Check sheet for the modelled part. Datum: model origin and axes. Units: mm. Give positions to 0.01 mm unless a question says otherwise; leave off trailing zeros. Order: outer loops, then holes, each group sorted by start corner. A loop starts at its lowest first (then second) coordinate and runs counter-clockwise, first axis right, second up. Notation, with made-up numbers: (-33.5, 8) -> (19.5, 8) arc R18 cw to (19.5, 27) -> close; hole circle Ø4 at (32, -34.5). An arc over 180 degrees is marked (long way). One line per question, with ' | ' between items.
```python
from build123d import *

# Parameters (mm, degrees)
SKETCH1_R           = 1.5
BOSS_EXTRUDE1_DEPTH = 2.5


with BuildPart() as part:
    # Sketch1 → Boss-Extrude1 (new, symmetric)
    with BuildSketch(Plane.XY):
        with BuildLine():
            Line((-30.46875, 2.5), (30.46875, 2.5))
            ThreePointArc((30.46875, 2.5), (32.96875, 0), (30.46875, -2.5))
            Line((30.46875, -2.5), (-30.46875, -2.5))
            ThreePointArc((-30.46875, -2.5), (-32.96875, 0), (-30.46875, 2.5))
        make_face()
        with Locations((-30.46875, 0)):
            Circle(SKETCH1_R, mode=Mode.SUBTRACT)
        with Locations((30.46875, 0)):
            Circle(SKETCH1_R, mode=Mode.SUBTRACT)
        with Locations((0.40625, 0)):
            Circle(SKETCH1_R, mode=Mode.SUBTRACT)
    extrude(amount=BOSS_EXTRUDE1_DEPTH, both=True)


solid = part.part
```
Q1. Section check A-A (z = 1.55). Enter the section's corners in (x, y), and give its area (3 significant figures).
Result sheet:
outline: (-30.47, -2.5) -> (30.47, -2.5) arc R2.5 ccw to (30.47, 2.5) -> (-30.47, 2.5) arc R2.5 ccw to start; hole circle Ø3 at (-30.47, 0); hole circle Ø3 at (0.41, 0); hole circle Ø3 at (30.47, 0) | area: 303 mm2
Q2. Depth check by flat-ended pin: pin 1 Ø2.5 at (x, y) = (-30.47, 0) entering from -Z. Enter the tip coordinate at first touch or a pass-through.
Result sheet:
pin 1: passes through
Q3. Section check B-B (y = 0). Enter the section's corners in (x, z).
Result sheet:
outline: (-32.97, -2.5) -> (-31.97, -2.5) -> (-31.97, 2.5) -> (-32.97, 2.5) -> close; (-28.97, -2.5) -> (-1.09, -2.5) -> (-1.09, 2.5) -> (-28.97, 2.5) -> close; (1.91, -2.5) -> (28.97, -2.5) -> (28.97, 2.5) -> (1.91, 2.5) -> close; (31.97, -2.5) -> (32.97, -2.5) -> (32.97, 2.5) -> (31.97, 2.5) -> close
Q4. Thickness scan on line 1 (X direction, y = 0.15, z = 0.85); line 2 (Y direction, x = 30.5, z = 1.4); line 3 (X direction, y = 0.8, z = 1.05). Record the ranges inside material, lowest first.
Result sheet:
line 1: x = -32.96 to -31.96, -28.98 to -1.09, 1.9 to 28.98, 31.96 to 32.96 | line 2: y = -2.5 to -1.5, 1.5 to 2.5 | line 3: x = -32.84 to -31.74, -29.2 to -0.86, 1.68 to 29.2, 31.74 to 32.84
Q5. Mould release check, pull along X, two halves, no side actions. Record for faces 1 (the face through (32.97, 0.05, 0.04)), 2 (the face through (-32.97, -0.05, 0.04)), 3 (the face through (0, -2.5, 0)), 4 (the face through (-31.967, 0.066, -0.035)): pulls with the +X half, pulls with the -X half, needs draft (parallel to the pull), parting line crosses it, or undercut.
Result sheet:
face 1: pulls with the +X half | face 2: pulls with the -X half | face 3: needs draft | face 4: undercut
